Print and shaded views of the part. All mm, measured from the part's lowest x, y and z. A direction names the side the tool comes from. Coordinates: 2 decimals unless noted, no trailing zeros. Loops run counter-clockwise (first coordinate to the right, second up) from the corner with the lowest first, then second, coordinate; pieces in that order, holes last.
1) Two-plate mould, pull along Y, no slides. Class the marked faces 5, 6 and 7: +Y half, -Y half, draft (parallel to the pull), parting line (faces both ways), or undercut.
2) Saw through at B-B, the plane x = 30. Write the cut outline in (y, z).
3) Saw through at D-D, the plane x = 84.5. Write the cut outline in (y, z), and give its area (3 significant figures).
4) Saw through at A-A, the plane y = 30. Write the cut outline in (x, z), and give its area (3 significant figures).
5) Saw through at C-C, the plane z = 25. Write the cut outline in (x, y).
6) Wall check: line 1 along Y through (x, z) = (30, 3); line 2 along X through (y, z) = (42.5, 9.5); line 3 along Z through (x, y) = (22.5, 33). Give the ranges that are in metal, low to high.
7) Pin check, flat tips, straight feed: pin 1 Ø6 at (y, z) = (17.5, 42) entering from -X; pin 2 Ø9 at (x, y) = (36.5, 31) entering from -Z; pin 3 Ø6 at (x, z) = (40.5, 29.5) entering from -Y; pin 4 Ø10 at (y, z) = (18.5, 13) entering from +X. Stop position of each tip, or through.
8) Which spindle directions (+Z, -Z, +X, -X, +Y, -Y) get a long thin tool onto all of the face, cutting with end or side? Do the marked faces 1, 2, 3 and 4. Say none if no direction does.
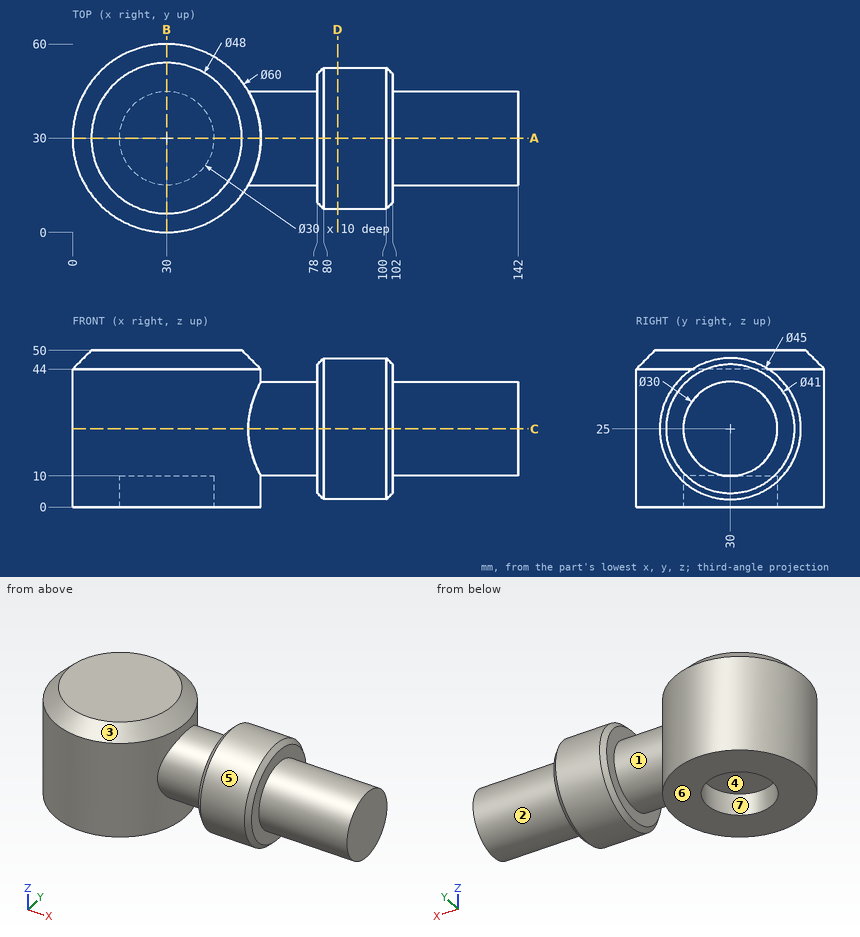
Data:
1. face 5: parting line
1. face 6: draft
1. face 7: undercut
2. outline: (0, 0) - (15, 0) - (15, 10) - (45, 10) - (45, 0) - (60, 0) - (60, 44) - (54, 50) - (6, 50) - (0, 44) - close
3. outline: circle Ø45 at (30, 25)
3. area: 1,590 mm2
4. outline: (0, 0) - (15, 0) - (15, 10) - (45, 10) - (45, 0) - (60, 0) - (60, 10) - (78, 10) - (78, 4.5) - (80, 2.5) - (100, 2.5) - (102, 4.5) - (102, 10) - (142, 10) - (142, 40) - (102, 40) - (102, 45.5) - (100, 47.5) - (80, 47.5) - (78, 45.5) - (78, 40) - (60, 40) - (60, 44) - (54, 50) - (6, 50) - (0, 44) - close
4. area: 5,480 mm2
5. outline: (55.98, 15) - (78, 15) - (78, 9.5) - (80, 7.5) - (100, 7.5) - (102, 9.5) - (102, 15) - (142, 15) - (142, 45) - (102, 45) - (102, 50.5) - (100, 52.5) - (80, 52.5) - (78, 50.5) - (78, 45) - (55.98, 45) arc R30 ccw (long way) to start
6. line 1: y = 0 to 15, 45 to 60
6. line 2: x = 2.73 to 21.71, 38.29 to 57.27, 78 to 102
6. line 3: z = 10 to 50
7. pin 1: stops at x = 1.54
7. pin 2: stops at z = 10
7. pin 3: stops at y = 0.95
7. pin 4: stops at x = 142
8. face 1: none
8. face 2: +X
8. face 3: +Z
8. face 4: -Z
